Read the model definition and answer for the solid it produces. Units are mm, in the model's axes. Face numbers are marked on the shaded views. A direction names the side the tool comes from. Coordinates: 2 decimals unless noted, no trailing zeros. Loops run counter-clockwise (first coordinate to the right, second up) from the corner with the lowest first, then second, coordinate; pieces in that order, holes last. Notation, with made-up numbers: M 21,46 L 44,46 A38 cw 44,84 Z; hole C -32,35.5 d11. An arc over 180 degrees is marked long. Use one line per item in the form item = value. Start each with the question number.
1. The part is cut by section A-A (x = 0). Give the vertices of the cut face in (y, z) (3 decimals), plus the area to 3 significant figures.
2. Flat-ended cylindrical pins translate along their axes: pin 1 (10 mm diameter, centred on x = -5.5, z = 1.5, fed in from +Y); pin 2 (1.9 mm diameter, centred on x = 0, y = 12, fed in from -Z). Find the tip coordinate at first contact, or state that the pin passes through.
3. The part is cut by section C-C (y = 12). Give the vertices of the cut face in (x, z) (3 decimals), plus the area to 3 significant figures.
4. The part is cut by section D-D (z = -14). Give the vertices of the cut face in (x, y).
5. Find the intervals of material crossed by probe 1 along Z at (x, y) = (-1.5, 16.5); probe 2 along Y at (x, z) = (-4, -19.5); probe 3 along Y at (x, z) = (0, -24.5) (3 decimals), in increasing order. Write a range as [from, to].
6. The part is cut by section B-B (y = 17). Give the vertices of the cut face in (x, z), plus the area to 3 significant figures.
7. A tool of negligible diameter and unlimited length cuts with its end or side. For the marked faces 1 and 2, from which of +Z, -Z, +X, -X, +Y, -Y can it reach the whole face along a straight path? Write none if from no direction.
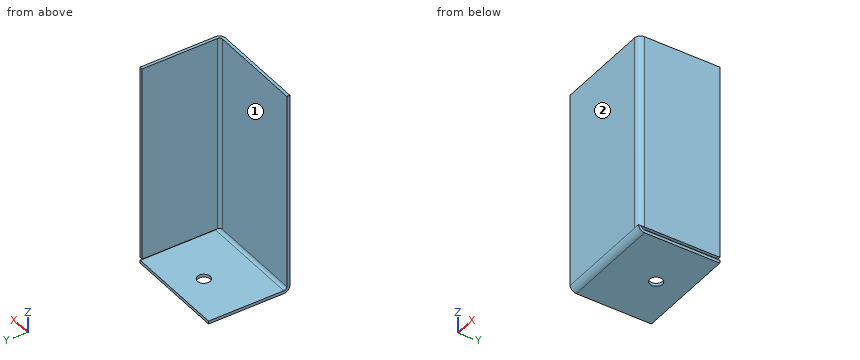
from build123d import *

# Parameters (mm, degrees)
SKETCH1_W                    = 25
SKETCH1_H                    = 50
BASE_FLANGE1_DEPTH           = 0.7366
EDGE_FLANGE1_STRIP_W         = 4.4196
EDGE_FLANGE1_STRIP_H         = 0.7366
EDGE_FLANGE1_STRIP_CUT_DEPTH = 25
EDGE_FLANGE1_DEPTH           = 25
EDGE_FLANGE1_PROFILE_W       = 25
EDGE_FLANGE1_PROFILE_H       = 18.5268
EDGE_FLANGE1_PROFILE_R       = 1.565
EDGE_FLANGE1_FLAT_DEPTH      = 0.7366
EDGE_FLANGE3_STRIP_W         = 4.4196
EDGE_FLANGE3_STRIP_H         = 0.7366
EDGE_FLANGE3_STRIP_CUT_DEPTH = 48.5268
EDGE_FLANGE3_DEPTH           = 48.5268


# Sheet-metal steps are written as plain solids
with BuildPart() as part:
    # Sketch1 → Base-Flange1 (new body)
    with BuildSketch(Plane(origin=(0, 0, 0), x_dir=(1, 0, 0), z_dir=(0, 1, 0))):
        Rectangle(SKETCH1_W, SKETCH1_H)
    extrude(amount=-BASE_FLANGE1_DEPTH)

    # Edge-Flange1 strip (across the edge) → Edge-Flange1 strip cut (cut)
    with BuildSketch(Plane(origin=(12.5, 0, -25), x_dir=(0, 0, 1), z_dir=(-1, 0, 0))):
        with Locations((-0.7366, -0.3683)):
            Rectangle(EDGE_FLANGE1_STRIP_W, EDGE_FLANGE1_STRIP_H)
    extrude(amount=EDGE_FLANGE1_STRIP_CUT_DEPTH, mode=Mode.SUBTRACT)

    # Edge-Flange1 bend section (across the edge) → Edge-Flange1 (add)
    with BuildSketch(Plane(origin=(12.5, 0, -25), x_dir=(0, 0, 1), z_dir=(-1, 0, 0))):
        with BuildLine():
            Line((0, 0.7366), (0.7366, 0.7366))
            ThreePointArc((0.7366, 0.7366), (0.952345145, 0.215745145), (1.4732, 0))
            Line((1.4732, 0), (1.4732, -0.7366))
            ThreePointArc((1.4732, -0.7366), (0.43149029, -0.30510971), (0, 0.7366))
        make_face()
    extrude(amount=EDGE_FLANGE1_DEPTH)

    # Edge-Flange1 profile (on flange) → Edge-Flange1 flat (add)
    with BuildSketch(Plane(origin=(0, 0, -25), x_dir=(-1, 0, 0), z_dir=(0, 0, -1))):
        with Locations((0, 10)):
            Rectangle(EDGE_FLANGE1_PROFILE_W, EDGE_FLANGE1_PROFILE_H)
        with Locations((0, 12)):
            Circle(EDGE_FLANGE1_PROFILE_R, mode=Mode.SUBTRACT)
    extrude(amount=-EDGE_FLANGE1_FLAT_DEPTH)

    # Edge-Flange3 strip (across the edge) → Edge-Flange3 strip cut (cut)
    with BuildSketch(Plane(origin=(12.5, 0, 25), x_dir=(-1, 0, 0), z_dir=(0, 0, -1))):
        with Locations((-0.7366, -0.3683)):
            Rectangle(EDGE_FLANGE3_STRIP_W, EDGE_FLANGE3_STRIP_H)
    extrude(amount=EDGE_FLANGE3_STRIP_CUT_DEPTH, mode=Mode.SUBTRACT)

    # Edge-Flange3 section (across the edge) → Edge-Flange3 (add)
    with BuildSketch(Plane(origin=(12.5, 0, 25), x_dir=(-1, 0, 0), z_dir=(0, 0, -1))):
        with BuildLine():
            Line((0, 0.7366), (0, 19.2634))
            Line((0, 19.2634), (0.7366, 19.2634))
            Line((0.7366, 19.2634), (0.7366, 0.7366))
            ThreePointArc((0.7366, 0.7366), (0.952345145, 0.215745145), (1.4732, 0))
            Line((1.4732, 0), (1.4732, -0.7366))
            ThreePointArc((1.4732, -0.7366), (0.43149029, -0.30510971), (0, 0.7366))
        make_face()
    extrude(amount=EDGE_FLANGE3_DEPTH)


solid = part.part
Computed values:
q1.outline = M -0.737,-23.527 A1.473 ccw 0.737,-25 L 10.435,-25 L 10.435,-24.263 L 0.737,-24.263 A0.737 cw 0,-23.527 L 0,25 L -0.737,25 Z; M 13.565,-25 L 19.263,-25 L 19.263,-24.263 L 13.565,-24.263 Z
q1.area = 48.4 mm²
q2.pin_1 = 0
q2.pin_2 = through
q3.outline = M -12.5,-25 L -1.565,-25 L -1.565,-24.263 L -12.5,-24.263 Z; M 1.565,-25 L 12.5,-25 L 12.5,-24.263 L 1.565,-24.263 Z; M 11.763,-23.527 L 12.5,-23.527 L 12.5,25 L 11.763,25 Z
q3.area = 51.9 mm²
q4.outline = M -12.5,-0.74 L 11.03,-0.74 A1.47 ccw 12.5,0.74 L 12.5,19.26 L 11.76,19.26 L 11.76,0.74 A0.74 cw 11.03,0 L -12.5,0 Z
q5.probe_1 = [-25, -24.26]
q5.probe_2 = [-0.74, 0]
q5.probe_3 = [-0.369, 10.435], [13.565, 19.263]
q6.outline = M -12.5,-25 L 12.5,-25 L 12.5,-24.26 L -12.5,-24.26 Z; M 11.76,-23.53 L 12.5,-23.53 L 12.5,25 L 11.76,25 Z
q6.area = 54.2 mm²
q7.face_1 = +Z, -X, +Y
q7.face_2 = +Z, -Z, +X, -X, -Y
